Can you work these out from the model? Positions are in its coordinate system, mm. Face numbers are marked on the shaded views. Coordinates: 2 decimals unless noted, no trailing zeros. Write each loop counter-clockwise with the first axis right and the second up, starting at its lowest first coordinate (ties: lowest second). Pieces come first, ordered by that corner, then holes. Notation, with made-up numbers: (48, 39) -> (95, 39) arc R24 ccw to (95, 70) -> close; hole circle Ø9 at (9.25, 84.5). An arc over 180 degrees is marked (long way). Answer as CSV lines item,"result". Start each with the question number.
```python
from build123d import *

# Parameters (mm, degrees)
SKETCH1_W            = 170
SKETCH1_H            = 82.55
BOSS_EXTRUDE1_DEPTH  = 5
SKETCH2_R            = 5.5
SKETCH2_R_2          = 3.025
BOSS_EXTRUDE2_DEPTH  = 5
SKETCH3_W            = 20
SKETCH3_H            = 15
BOSS_EXTRUDE3_DEPTH  = 5
FILLET1_R            = 6
M4_CLEARANCE_HOLE1_D = 4.5


with BuildPart() as part:
    # Sketch1 → Boss-Extrude1 (new body)
    with BuildSketch(Plane.XY):
        Rectangle(SKETCH1_W, SKETCH1_H)
    extrude(amount=BOSS_EXTRUDE1_DEPTH)

    # Sketch2 → Boss-Extrude2 (add)
    with BuildSketch(Plane.XY.offset(5)):
        with Locations((65, 25)):
            Circle(SKETCH2_R)
        with Locations((65, 25)):
            Circle(SKETCH2_R_2, mode=Mode.SUBTRACT)
        with Locations((8.25, 25)):
            Circle(SKETCH2_R)
        with Locations((8.25, 25)):
            Circle(SKETCH2_R_2, mode=Mode.SUBTRACT)
        with Locations((-65, 25)):
            Circle(SKETCH2_R)
        with Locations((-65, 25)):
            Circle(SKETCH2_R_2, mode=Mode.SUBTRACT)
        with Locations((-65, -25)):
            Circle(SKETCH2_R)
        with Locations((-65, -25)):
            Circle(SKETCH2_R_2, mode=Mode.SUBTRACT)
        with Locations((8.25, -25)):
            Circle(SKETCH2_R)
        with Locations((8.25, -25)):
            Circle(SKETCH2_R_2, mode=Mode.SUBTRACT)
        with Locations((65, -25)):
            Circle(SKETCH2_R)
        with Locations((65, -25)):
            Circle(SKETCH2_R_2, mode=Mode.SUBTRACT)
    extrude(amount=BOSS_EXTRUDE2_DEPTH)

    # Sketch3 → Boss-Extrude3 (add)
    with BuildSketch(Plane.XY.offset(5)):
        Polygon((-65, 56.275), (-85, 41.275), (-65, 41.275), align=None)
        Polygon((-85, 56.275), (-85, 41.275), (-65, 56.275), align=None)
        with Locations((75, -48.775)):
            Rectangle(SKETCH3_W, SKETCH3_H)
    extrude(amount=-BOSS_EXTRUDE3_DEPTH)

    # Fillet1
    fillet1_edges = [part.edges().sort_by_distance(p)[0] for p in [
        (-85, 56.275, 2.5),
        (-65, 56.275, 2.5),
        (-65, 41.275, 2.5),
        (65, -56.275, 2.5),
        (65, -41.275, 2.5),
        (85, -56.275, 2.5),
        (-85, -41.275, 2.5),
        (85, 41.275, 2.5),
    ]]
    fillet(fillet1_edges, radius=FILLET1_R)

    # M4 Clearance Hole1 (through all)
    with Locations(Plane.XY.offset(5)):
        with Locations((-75, 48.775), (75, -48.775)):
            Hole(M4_CLEARANCE_HOLE1_D / 2)


solid = part.part
```
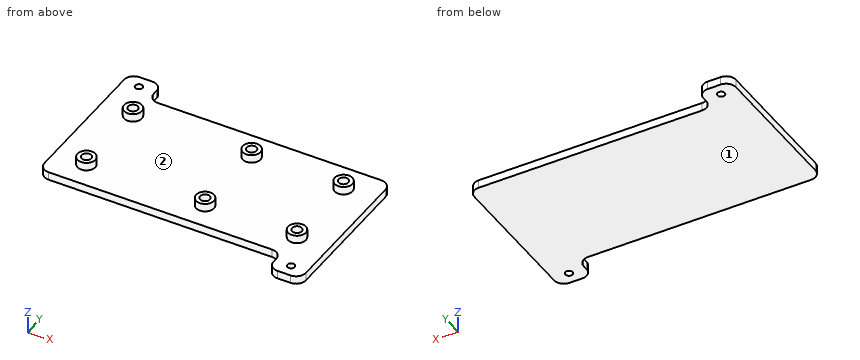
Q1. For pin 1 (1.5 mm diameter, centred on x = -15.5, y = 16, fed in from +Z); pin 2 (1.5 mm diameter, centred on x = -11, z = 2.5, fed in from -Y) (3 decimals); pin 3 (5.5 mm diameter, centred on x = -1, z = 2.5, fed in from +Y) (3 decimals), each with a flat end and sliding along its axis, tell me the tip position at first contact or that it passes through.
Q2. Imagine slicing it at D-D (y = 25). Write out the boundary of the cut face in (x, z) (3 decimals).
Q3. I need wall thicknesses on L1, parallel to Y at x = 8.25, z = 8.35 (3 decimals); L2, parallel to Y at x = -75, z = 2.2 (3 decimals); L3, parallel to Y at x = 21.5, z = 1.25 (3 decimals). Which ranges of each line are inside material? Lowest first, please.
Q4. Imagine slicing it at A-A (z = 7.25). State how many separate pieces and enclosed holes the cut face has, then the cut area to 3 significant figures.
Q5. Imagine slicing it at B-B (x = 75). Write out the boundary of the cut face in (y, z) (3 decimals).
Q6. If we mould it in two halves opening along X, with no side actions, what happens to the marked faces 1 and 2? For each: released by +X, released by -X, zero draft, split by the parting line, or undercut.
Q7. Imagine slicing it at C-C (x = 8.25). Write out the boundary of the cut face in (y, z) (3 decimals).
Entries:
1,pin 1,"z = 5"
1,pin 2,"y = -41.275"
1,pin 3,"y = 41.275"
2,outline,"(-85, 0) -> (85, 0) -> (85, 5) -> (70.5, 5) -> (70.5, 10) -> (68.025, 10) -> (68.025, 5) -> (61.975, 5) -> (61.975, 10) -> (59.5, 10) -> (59.5, 5) -> (13.75, 5) -> (13.75, 10) -> (11.275, 10) -> (11.275, 5) -> (5.225, 5) -> (5.225, 10) -> (2.75, 10) -> (2.75, 5) -> (-59.5, 5) -> (-59.5, 10) -> (-61.975, 10) -> (-61.975, 5) -> (-68.025, 5) -> (-68.025, 10) -> (-70.5, 10) -> (-70.5, 5) -> (-85, 5) -> close"
3,L1,"-30.5 to -28.025, -21.975 to -19.5, 19.5 to 21.975, 28.025 to 30.5"
3,L2,"-41.275 to 46.525, 51.025 to 56.275"
3,L3,"-41.275 to 41.275"
4,separate pieces,"6"
4,enclosed holes,"6"
4,area,"398 mm2"
5,outline,"(-56.275, 0) -> (-51.025, 0) -> (-51.025, 5) -> (-56.275, 5) -> close; (-46.525, 0) -> (41.275, 0) -> (41.275, 5) -> (-46.525, 5) -> close"
6,face 1,"zero draft"
6,face 2,"undercut"
7,outline,"(-41.275, 0) -> (41.275, 0) -> (41.275, 5) -> (30.5, 5) -> (30.5, 10) -> (28.025, 10) -> (28.025, 5) -> (21.975, 5) -> (21.975, 10) -> (19.5, 10) -> (19.5, 5) -> (-19.5, 5) -> (-19.5, 10) -> (-21.975, 10) -> (-21.975, 5) -> (-28.025, 5) -> (-28.025, 10) -> (-30.5, 10) -> (-30.5, 5) -> (-41.275, 5) -> close"
